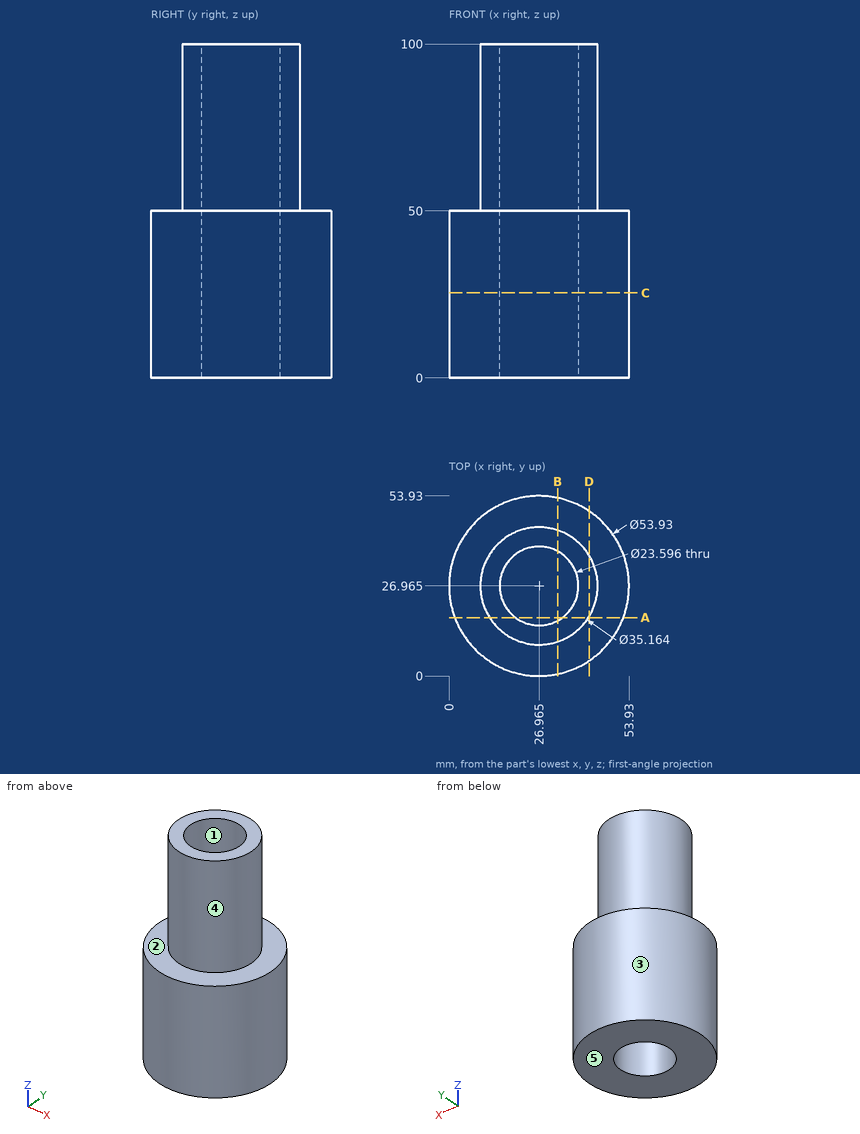
For this review, use the dimensioned drawing (mm, ordinates from the lowest corner) and the shaded views. A direction names the side the tool comes from. Round coordinates to 2 decimals unless told otherwise and drop trailing zeros. Order: outer loops, then holes, each group sorted by start corner. A loop starts at its lowest first (then second) coordinate and runs counter-clockwise, first axis right, second up. Notation, with made-up numbers: (77, -11.75) -> (99, -11.75) arc R10 cw to (99, -6.75) -> close; hole circle Ø8 at (38.5, 39.5). An arc over 180 degrees is marked (long way). Use CSV: the item, a comma, the result in double quotes. Start each with the question number.
(1) Wall thickness on probe 1 along Y at (x, z) = (27.5, 94); probe 2 along Z at (x, y) = (46.5, 21); probe 3 along X at (y, z) = (34, 13) (1 decimal): over which ranges is each line inside the solid? List them lowest first. Write a range as from..to.
(2) Consider section C-C on z = 25.5. Write out the cut boundary in (x, y) (1 decimal), and give its area (3 significant figures).
(3) Tool access review of the marked faces 4 and 5: name each direction out of +Z, -Z, +X, -X, +Y, -Y from which nothing blocks a thin tool from reaching the whole face with its end or side.
(4) Insertion check: pin 1 (6 mm diameter, centred on y = 15.5, z = 78, fed in from +X) (1 decimal); pin 2 (3 mm diameter, centred on y = 17.5, z = 31, fed in from +X); pin 3 (4 mm diameter, centred on y = 20, z = 14.5, fed in from -X). Each pin has a flat end and moves straight along its axis. Give the tip position at first contact, or say it passes through.
(5) Consider section B-B on x = 32.5. Write out the cut boundary in (y, z) (1 decimal).
(6) Consider section A-A on y = 17.5. Write out the cut boundary in (x, z).
(7) Consider section D-D on x = 42. Write out the cut boundary in (y, z).
(8) Mouldability with a two-part tool opening along Y and no side actions: class the marked faces 1, 2 and 3 as pulls with the +Y half, pulls with the -Y half, needs draft (parallel to the pull), parting line crosses it, or undercut.
Responses:
1,probe 1,"9.39..15.18, 38.75..44.54"
1,probe 2,"0..50"
1,probe 3,"0.9..17.5, 36.4..53"
2,outline,"circle Ø53.9 at (27, 27); hole circle Ø23.6 at (27, 27)"
2,area,"1,850 mm²"
3,face 4,"+Z"
3,face 5,"-Z, +X, -X, +Y, -Y"
4,pin 1,"x = 42.4"
4,pin 2,"x = 52.73"
4,pin 3,"x = 0.46"
5,outline,"(0.6, 0) -> (16.5, 0) -> (16.5, 100) -> (10.3, 100) -> (10.3, 50) -> (0.6, 50) -> close; (37.4, 0) -> (53.4, 0) -> (53.4, 50) -> (43.7, 50) -> (43.7, 100) -> (37.4, 100) -> close"
6,outline,"(1.72, 0) -> (19.92, 0) -> (19.92, 100) -> (12.15, 100) -> (12.15, 50) -> (1.72, 50) -> close; (34.01, 0) -> (52.21, 0) -> (52.21, 50) -> (41.78, 50) -> (41.78, 100) -> (34.01, 100) -> close"
7,outline,"(4.58, 0) -> (49.35, 0) -> (49.35, 50) -> (36.08, 50) -> (36.08, 100) -> (17.85, 100) -> (17.85, 50) -> (4.58, 50) -> close"
8,face 1,"undercut"
8,face 2,"needs draft"
8,face 3,"parting line crosses it"
